from build123d import *

# Parameters (mm, degrees)
SKETCH1_R           = 22.5
BOSS_EXTRUDE1_DEPTH = 10
CUT_EXTRUDE1_REACH  = 12
SKETCH2_R           = 18.1
SKETCH3_R           = 3.275


with BuildPart() as part:
    # Sketch1 → Boss-Extrude1 (new body)
    with BuildSketch(Plane.XY):
        Circle(SKETCH1_R)
    extrude(amount=BOSS_EXTRUDE1_DEPTH)

    # Sketch2 → Cut-Extrude1 (cut, up to next)
    with BuildSketch(Plane.XY.offset(10), mode=Mode.PRIVATE) as cut_extrude1_sk1:
        Circle(SKETCH2_R)
    cut_extrude1_tool1 = extrude(cut_extrude1_sk1.sketch, amount=-CUT_EXTRUDE1_REACH, mode=Mode.PRIVATE) & part.part
    add(cut_extrude1_tool1.solids().sort_by_distance((0, 0, 10))[0], mode=Mode.SUBTRACT)

    # Sketch3 → Cut-Revolve1 (revolve, cut)
    with BuildSketch(Plane(origin=(0, 0, 0), x_dir=(1, 0, 0), z_dir=(0, 1, 0))):
        with Locations((-24, -5)):
            Circle(SKETCH3_R)
    revolve(axis=Axis((0, 0, -18.462767292), (0, 0, 1)), mode=Mode.SUBTRACT)


solid = part.part
Source: CAD feature listing. Evaluate the final solid. Frame: model axes, mm. Give positions to 0.01 mm unless a question says otherwise; leave off trailing zeros. Write each loop counter-clockwise with the first axis right and the second up, starting at its lowest first coordinate (ties: lowest second). Pieces come first, ordered by that corner, then holes. Notation, with made-up numbers: (-12, -21.5) -> (-1, -21.5) arc R21 cw to (-1, -12.5) -> close; hole circle Ø8 at (63, -33). An arc over 180 degrees is marked (long way). Write item = value, one per line.
Q1. First-contact query: pin 1 (3 mm diameter, centred on x = 3, z = 1, fed in from +Y); pin 2 (3 mm diameter, centred on y = 8, z = 3.5, fed in from +X); pin 3 (1.5 mm diameter, centred on y = -14.5, z = 1.5, fed in from -X). Flat tips, straight axial feed; report the tip coordinate or a pass-through.
Here are the results:
pin_1 = 22.45
pin_2 = 21.22
pin_3 = -17.81
Q2. Cut plane C-C on z = 9. Return loops of the section in (x, y), then the cut area to 3 significant figures.
Here are the results:
outline = circle Ø45 at (0, 0); hole circle Ø36.2 at (0, 0)
area = 561 mm²
Q3. Cut plane A-A on x = 0. Return loops of the section in (y, z) (3 decimals), then the cut area to 3 significant figures.
Here are the results:
outline = (-22.5, 0) -> (-18.1, 0) -> (-18.1, 10) -> (-22.5, 10) -> (-22.5, 7.911) arc R3.275 cw to (-22.5, 2.089) -> close; (18.1, 0) -> (22.5, 0) -> (22.5, 2.089) arc R3.275 cw to (22.5, 7.911) -> (22.5, 10) -> (18.1, 10) -> close
area = 73.2 mm²
Q4. Line query: line 1 (X direction, y = 8, z = 7.75); line 2 (Z direction, x = 21, y = 2); line 3 (X direction, y = 5.5, z = 6.25). Output: solid intervals per line, ascending. Write a range as from..to.
Here are the results:
line_1 = -20.73..-16.24, 16.24..20.73
line_2 = 0..3.49, 6.51..10
line_3 = -20.24..-17.24, 17.24..20.24
Q5. Mould query, pull axis Y, two halves, no side actions, for faces 1 (the face through (10.382, -19.961, 1.03)), 2 (the face through (1.6, 18.4, 0)), 3 (the face through (17.264, 5.437, 5.07)). Classes: +Y half, -Y half, draft (parallel to the pull), parting line (faces both ways), or undercut.
Here are the results:
face_1 = parting line
face_2 = draft
face_3 = undercut
